Could you check a few things on this model? Use its own coordinates, in mm. Face numbers are marked on the shaded views. Give positions to 0.01 mm unless a question says otherwise; leave off trailing zeros. Order: outer loops, then holes, each group sorted by start corner. A loop starts at its lowest first (then second) coordinate and runs counter-clockwise, first axis right, second up.
Autodesk Inventor part; units mm, degrees
ref_plane "YZ Plane" through (0, 0, 0) normal (1, 0, 0) x (0, 1, 0)
ref_plane "XZ Plane" through (0, 0, 0) normal (0, 1, 0) x (-1, 0, 0)
ref_plane "XY Plane" through (0, 0, 0) normal (0, 0, 1) x (1, 0, 0)
sketch "スケッチ1" plane through (0, 0, 0) normal (0, 0, 1) x (1, 0, 0)
  line L0 (-26.2, 56.2) -> (26.2, 56.2)
  line L1 (26.2, 56.2) -> (26.2, -56.2)
  line L2 (26.2, -56.2) -> (-26.2, -56.2)
  line L3 (-26.2, -56.2) -> (-26.2, 56.2)
  line L4 (-26.2, 56.2) -> (26.2, -56.2) construction
  line L5 (26.2, 56.2) -> (-26.2, -56.2) construction
  line L6 (-25.2, 55.2) -> (25.2, 55.2)
  line L7 (25.2, 55.2) -> (25.2, -55.2)
  line L8 (25.2, -55.2) -> (-25.2, -55.2)
  line L9 (-25.2, -55.2) -> (-25.2, 55.2)
  line L10 (-25.2, 55.2) -> (25.2, -55.2) construction
  line L11 (25.2, 55.2) -> (-25.2, -55.2) construction
  line L12 (-25, 55) -> (25, 55) construction
  line L13 (25, 55) -> (25, -55) construction
  line L14 (25, -55) -> (-25, -55) construction
  line L15 (-25, -55) -> (-25, 55) construction
  line L16 (-25, 55) -> (25, -55) construction
  line L17 (25, 55) -> (-25, -55) construction
  line L18 (-26.25, 56.25) -> (26.25, 56.25) construction
  line L19 (26.25, 56.25) -> (26.25, -56.25) construction
  line L20 (26.25, -56.25) -> (-26.25, -56.25) construction
  line L21 (-26.25, -56.25) -> (-26.25, 56.25) construction
  line L22 (-26.25, 56.25) -> (26.25, -56.25) construction
  line L23 (26.25, 56.25) -> (-26.25, -56.25) construction
  circle A0 centre (-21, 51) radius 1.75
  circle A1 centre (-21, -28) radius 1.75
  line L24 (0, 56.25) -> (0, -56.25) construction
  circle A2 centre (21, 51) radius 1.75
  circle A3 centre (21, -28) radius 1.75
  arc A4 (-21, -32) -> (-21, -24) centre (-21, -28) ccw
  line L25 (-21, 47) -> (-25.2, 47)
  line L26 (-17, 51) -> (-17, 55.2)
  arc A5 (-21, 47) -> (-17, 51) centre (-21, 51) ccw
  line L27 (-21, -24) -> (-25.2, -24)
  line L28 (-21, -32) -> (-25.2, -32)
  arc A6 (21, -24) -> (21, -32) centre (21, -28) ccw
  line L29 (21, 47) -> (25.2, 47)
  line L30 (17, 51) -> (17, 55.2)
  arc A7 (17, 51) -> (21, 47) centre (21, 51) ccw
  line L31 (21, -24) -> (25.2, -24)
  line L32 (21, -32) -> (25.2, -32)
  line L33 (25.2, -53.2) -> (25.2, -38.2)
  line L34 (25.2, -38.2) -> (10.2, -38.2)
  line L35 (25.2, -53.2) -> (10.2, -53.2)
  line L36 (10.2, -53.2) -> (10.2, -38.2)
  line L37 (-22.2, -56.2) -> (-22.2, -55.2)
  line L38 (6.8, -56.2) -> (6.8, -55.2)
  point P0 (0, 0)
  point P1 (-25.2, -38.2)
  dimension "d0" = 50
  dimension "d1" = 110
  dimension "d2" = 0.2
  dimension "d4" = 0.2
  dimension "d8" = 1
  dimension "d10" = 1
  dimension "d11" = 112.5
  dimension "d12" = 0.05
  dimension "d13" = 0.05
  dimension "d14" = 52.5
  dimension "d15" = 3.5
  dimension "d16" = 4
  dimension "d17" = 4
  dimension "d18" = 3.5
  dimension "d19" = 4
  dimension "d20" = 83
  dimension "d22" = 8
  dimension "d31" = 4
  dimension "d33" = 15
  dimension "d34" = 15
  dimension "d36" = 2
  dimension "d37" = 29
  dimension "d38" = 4
extrude "押し出し1" add sketch "スケッチ1" along normal blind 4.8 contours L0 L1 L2 L38 L8 L7 L6 L9 L37 L3
extrude "押し出し2" add sketch "スケッチ1" against normal blind 1 contours L0 L1 L2 L38 L8 L7 L6 L9 L37 L3 | L37 L8 L38 L2 | L8 L9 L28 A4 L27 L25 A5 L26 L6 L30 A7 L29 L7 L31 A6 L32 L34 L36 L35 | L9 L27 A4 L28 | L9 L6 L26 A5 L25 | L32 A6 L31 L7 | L29 A7 L30 L6 L7
extrude "押し出し3" add sketch "スケッチ1" along normal blind 3.6 contours L9 L27 A4 L28 | L9 L6 L26 A5 L25 | L32 A6 L31 L7 | L29 A7 L30 L6 L7
fillet "フィレット1" radius 1 4 edges at (-26.2, -56.2, 1.9) (26.2, -56.2, 1.9) (26.2, 56.2, 1.9) (-26.2, 56.2, 1.9)
fillet "フィレット2" radius 1 28 edges at (-25.2, 47, 1.8) (-17, 55.2, 1.8) (-25.2, 11.5, 0) (-18.1716, 48.1716, 0) (-17, 53.1, 0) (-23.1, 47, 0) (0, 55.2, 0) (17, 53.1, 0) (23.1, 47, 0) (18.1716, 48.1716, 0) (17, 55.2, 1.8) (25.2, 47, 1.8) (25.2, 11.5, 0) (25.2, -32, 1.8) (23.1, -24, 0) (23.1, -32, 0) (17, -28, 0) (-23.1, -32, 0) (-23.1, -24, 0) (-17, -28, 0) (16, -55.2, 0) (-23.7, -55.2, 0) (-25.2, -43.6, 0) (-25.2, -32, 1.8) (-25.2, -24, 1.8) (25.2, -24, 1.8) (-22.2, -55.7, 0) (6.8, -55.7, 0)
fillet "フィレット4" radius 2 4 edges at (10.2, -38.2, -0.5) (10.2, -53.2, -0.5) (25.2, -53.2, -0.5) (25.2, -38.2, -0.5)
equation "\"d4\" = d2"
equation "\"d13\" = d12"
equation "\"d17\" = d16"
equation "\"d18\" = d15"
equation "\"d19\" = d17"
equation "\"d22\" = 2 * d31"
properties part number "J120_cover" material "アセタール樹脂、黒"
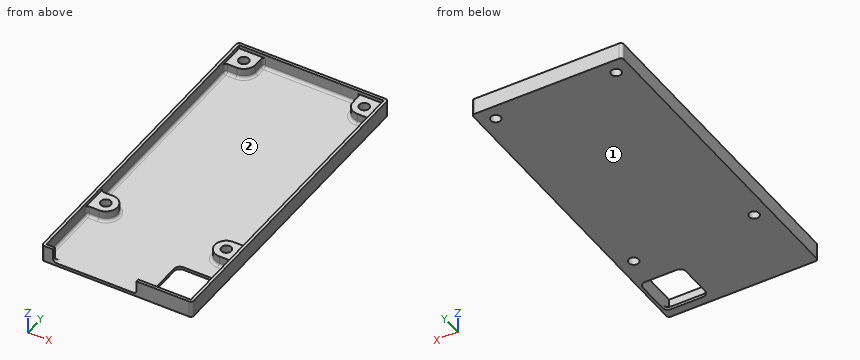
Item 1: For pin 1 (1 mm diameter, centred on x = -2, z = 2.5, fed in from -Y); pin 2 (4.5 mm diameter, centred on x = -21, y = 51, fed in from -Z); pin 3 (3 mm diameter, centred on x = -21, y = -28, fed in from -Z); pin 4 (15 mm diameter, centred on x = 4.5, y = 23.5, fed in from +Z), each with a flat end and sliding along its axis, tell me the tip position at first contact or that it passes through.
Findings:
pin 1: stops at y = 55.2
pin 2: stops at z = -1
pin 3: passes through
pin 4: stops at z = 0
Item 2: Imagine slicing it at C-C on x = 8. List the corners of the cut face in (y, z) for me.
Findings:
outline: (-56.2, -1) - (56.2, -1) - (56.2, 4.8) - (55.2, 4.8) - (55.2, 1) arc R1 cw to (54.2, 0) - (-54.2, 0) arc R1 cw to (-55.2, 1) - (-55.2, 4.8) - (-56.2, 4.8) - close
Item 3: Imagine slicing it at D-D on z = 2.2. Give the number of separate pieces and of enclosed holes in the cut face, then the cut area to 3 significant figures.
Findings:
separate pieces: 1
enclosed holes: 4
area: 504 mm2
Item 4: We'd pull the mould along Y, two halves only. Please class the marked faces 1 and 2: +Y half, -Y half, draft (parallel to the pull), parting line (faces both ways), or undercut.
Findings:
face 1: draft
face 2: undercut
Item 5: Imagine slicing it at A-A on x = 14. List the corners of the cut face in (y, z) for me.
Findings:
outline: (-56.2, -1) - (-53.2, -1) - (-53.2, 0) - (-54.2, 0) arc R1 cw to (-55.2, 1) - (-55.2, 4.8) - (-56.2, 4.8) - close; (-38.2, -1) - (56.2, -1) - (56.2, 4.8) - (55.2, 4.8) - (55.2, 1) arc R1 cw to (54.2, 0) - (-38.2, 0) - close
Item 6: Please list where these lines run through material, in increasing order: line 1 along Y through (x, z) = (21, 1.9); line 2 along X through (y, z) = (7.5, 4.2); line 3 along Y through (x, z) = (-21, 2.2).
Findings:
line 1: y = -56.2 to -55.2, -32 to -29.75, -26.25 to -24, 47 to 49.25, 52.75 to 56.2
line 2: x = -26.2 to -25.2, 25.2 to 26.2
line 3: y = -32 to -29.75, -26.25 to -24, 47 to 49.25, 52.75 to 56.2
Item 7: Imagine slicing it at B-B on y = -28. List the corners of the cut face in (x, z) for me, then the cut area to 3 significant figures.
Findings:
outline: (-26.2, -1) - (-22.75, -1) - (-22.75, 3.6) - (-25.2, 3.6) - (-25.2, 4.8) - (-26.2, 4.8) - close; (-19.25, -1) - (19.25, -1) - (19.25, 3.6) - (17, 3.6) - (17, 1) arc R1 cw to (16, 0) - (-16, 0) arc R1 cw to (-17, 1) - (-17, 3.6) - (-19.25, 3.6) - close; (22.75, -1) - (26.2, -1) - (26.2, 4.8) - (25.2, 4.8) - (25.2, 3.6) - (22.75, 3.6) - close
area: 89.3 mm2
